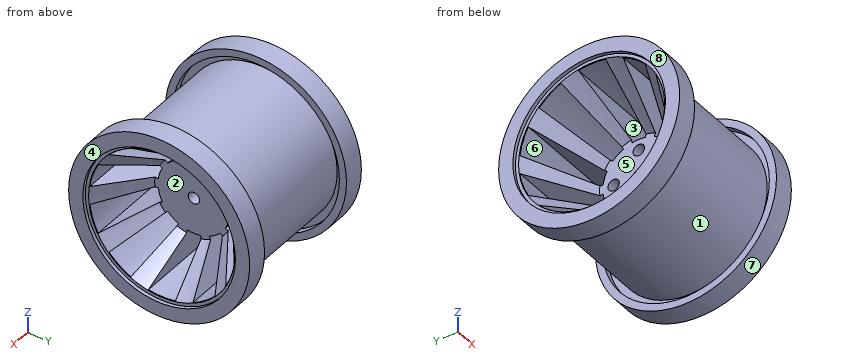
from build123d import *

# Parameters (mm, degrees)
SKETCH027_R        = 25.4
PAD009_DEPTH       = 22.5
POCKET015_DEPTH    = 214.544859
POLARPATTERN_COUNT = 10
SKETCH029_R        = 1.6
POCKET016_DEPTH    = 45.001
SKETCH030_R        = 21.4
POCKET017_DEPTH    = 1
SKETCH_R           = 21.4
POCKET_DEPTH       = 1
SKETCH031_R        = 10.1
POCKET018_DEPTH    = 19
SKETCH069_R        = 1.6
POCKET040_DEPTH    = 8
SKETCH035_R        = 10.1
POCKET020_DEPTH    = 13


with BuildPart() as part:
    # Sketch027 → Pad009 (new body, symmetric)
    with BuildSketch(Plane.YZ):
        Circle(SKETCH027_R)
    extrude(amount=PAD009_DEPTH, both=True)

    # Sketch028 (on Face3 of Pad009) → Pocket015 (cut, through all)
    with BuildSketch(Plane.YZ.offset(22.5)):
        with BuildLine():
            ThreePointArc((1.865103, 9.926298), (0, 10.1), (-1.865103, 9.926298))
            Line((-1.865103, 9.926298), (-3.806742, 20.041674))
            ThreePointArc((3.806742, 20.041674), (0, 20.4), (-3.806742, 20.041674))
            Line((3.806742, 20.041674), (1.865103, 9.926298))
        make_face()
    pocket015 = extrude(amount=-POCKET015_DEPTH, mode=Mode.SUBTRACT)

    # PolarPattern: Pocket015 ×10 about axis
    polarpattern_axis = Axis((22.5, 0, 0), (1, 0, 0))
    for i in range(1, POLARPATTERN_COUNT):
        add(pocket015.rotate(polarpattern_axis, i * 360 / POLARPATTERN_COUNT), mode=Mode.SUBTRACT)

    # Sketch033 → Groove (revolve, cut)
    with BuildSketch(Plane.XZ):
        Polygon((-16.5, 25.4), (16.5, 25.4), (16.5, 23.4), (18.5, 23.4), (18.5, 21.4), (-18.5, 21.4), (-18.5, 23.4), (-16.5, 23.4), align=None)
    revolve(axis=Axis((0, 0, 0), (1, 0, 0)), mode=Mode.SUBTRACT)

    # Sketch029 (on Face3 of PolarPattern) → Pocket016 (cut, through all)
    with BuildSketch(Plane.YZ.offset(22.5)):
        Circle(SKETCH029_R)
    extrude(amount=-POCKET016_DEPTH, mode=Mode.SUBTRACT)

    # Sketch030 (on Face2 of Pocket016) → Pocket017 (cut)
    with BuildSketch(Plane(origin=(-22.5, 0, 0), x_dir=(0, 1, 0), z_dir=(-1, 0, 0))):
        Circle(SKETCH030_R)
    extrude(amount=-POCKET017_DEPTH, mode=Mode.SUBTRACT)

    # Sketch (on Face50 of Pocket017) → Pocket (cut)
    with BuildSketch(Plane.YZ.offset(22.5)):
        Circle(SKETCH_R)
    extrude(amount=-POCKET_DEPTH, mode=Mode.SUBTRACT)

    # Sketch031 (on Face6 of Pocket017) → Pocket018 (cut)
    with BuildSketch(Plane(origin=(-21.5, 0, 0), x_dir=(0, 1, 0), z_dir=(-1, 0, 0))):
        Circle(SKETCH031_R)
    extrude(amount=-POCKET018_DEPTH, mode=Mode.SUBTRACT)

    # Sketch069 (on Face52 of Pocket018) → Pocket040 (cut)
    with BuildSketch(Plane(origin=(-2.5, 0, 0), x_dir=(0, 1, 0), z_dir=(-1, 0, 0))):
        with Locations((-7.071068, 0)):
            Circle(SKETCH069_R)
        with Locations((0, 7.071068)):
            Circle(SKETCH069_R)
        with Locations((7.071068, 0)):
            Circle(SKETCH069_R)
        with Locations((0, -7.071068)):
            Circle(SKETCH069_R)
    extrude(amount=-POCKET040_DEPTH, mode=Mode.SUBTRACT)

    # Sketch035 (on Face50 of Pocket040) → Pocket020 (cut)
    with BuildSketch(Plane.YZ.offset(21.5)):
        Circle(SKETCH035_R)
    extrude(amount=-POCKET020_DEPTH, mode=Mode.SUBTRACT)

    # Cone → Cone (revolve, cut)
    with BuildSketch(Plane(origin=(8.5, 0, 0), x_dir=(0, 1, 0), z_dir=(0, 0, -1))):
        Polygon((0, 0), (11, 0), (20.5, 13), (0, 13), align=None)
    revolve(axis=Axis((8.5, 0, 0), (1, 0, 0)), mode=Mode.SUBTRACT)

    # Cone001 → Cone001 (revolve, cut)
    with BuildSketch(Plane(origin=(-2.5, 0, 0), x_dir=(0, 1, 0), z_dir=(0, 0, 1))):
        Polygon((0, 0), (11, 0), (20.5, 19), (0, 19), align=None)
    revolve(axis=Axis((-2.5, 0, 0), (-1, 0, 0)), mode=Mode.SUBTRACT)


with BuildPart() as part_1:
    # Body006 placement: moved
    add(part.part.moved(Location((7.1, 0, 0))))


solid = part_1.part
Input: part model. Units: mm. Frame: model coordinates. Face numbers are marked on the shaded views. A direction names the side the tool comes from. Round coordinates to 2 decimals unless told otherwise and drop trailing zeros. Use a Markdown table: item, result.
1. Mould query, pull axis Z, two halves, no side actions, for the marked faces 6, 7 and 8. Classes: +Z half, -Z half, draft (parallel to the pull), parting line (faces both ways), or undercut.
Evaluation:
| item | result |
|---|---|
| face 6 | undercut |
| face 7 | parting line |
| face 8 | draft |
2. Material intervals for probe 1 along Z at (x, y) = (28, 0); probe 2 along Z at (x, y) = (9, 0); probe 3 along Y at (x, z) = (-9.8, 0), sorted ascending.
Evaluation:
| item | result |
|---|---|
| probe 1 | -25.4 to -20.4, 20.4 to 25.4 |
| probe 2 | -21.4 to -20.4, -10.1 to -8.67, -5.47 to -1.6, 1.6 to 5.47, 8.67 to 10.1, 20.4 to 21.4 |
| probe 3 | -25.4 to -23.4, -21.4 to -18.2, 18.2 to 21.4, 23.4 to 25.4 |
3. First-contact query: pin 1 (6 mm diameter, centred on x = 18.5, y = -13, fed in from +Z); pin 2 (4 mm diameter, centred on y = -9, z = -5, fed in from -X); pin 3 (2.5 mm diameter, centred on y = -6.5, z = -0.5, fed in from -X). Flat tips, straight axial feed; report the tip coordinate or a pass-through.
Evaluation:
| item | result |
|---|---|
| pin 1 | z = 18.92 |
| pin 2 | x = 2.01 |
| pin 3 | x = 4.6 |
4. Section A-A on y = 0. State how many separate pieces and enclosed holes the cut face has, then the cut area to 3 significant figures.
Evaluation:
| item | result |
|---|---|
| separate pieces | 4 |
| enclosed holes | 0 |
| area | 302 mm^2 |
5. Access query for the marked faces 1, 2, 3, 4 and 5. Directions: +Z, -Z, +X, -X, +Y, -Y. A direction counts if a zero-diameter tool reaches every point of the face in a straight line with its end or side. Return the directions, or none.
Evaluation:
| item | result |
|---|---|
| face 1 | none |
| face 2 | +X |
| face 3 | +X, -X |
| face 4 | +Z, -Z, +X, +Y, -Y |
| face 5 | -X |
